The drawing under review shows one solid part. Ordinate dimensions are in mm from its lowest x, y, z. A direction names the side the tool comes from. Give positions to 0.01 mm unless a question says otherwise; leave off trailing zeros. Loops run counter-clockwise (first coordinate to the right, second up) from the corner with the lowest first, then second, coordinate; pieces in that order, holes last.
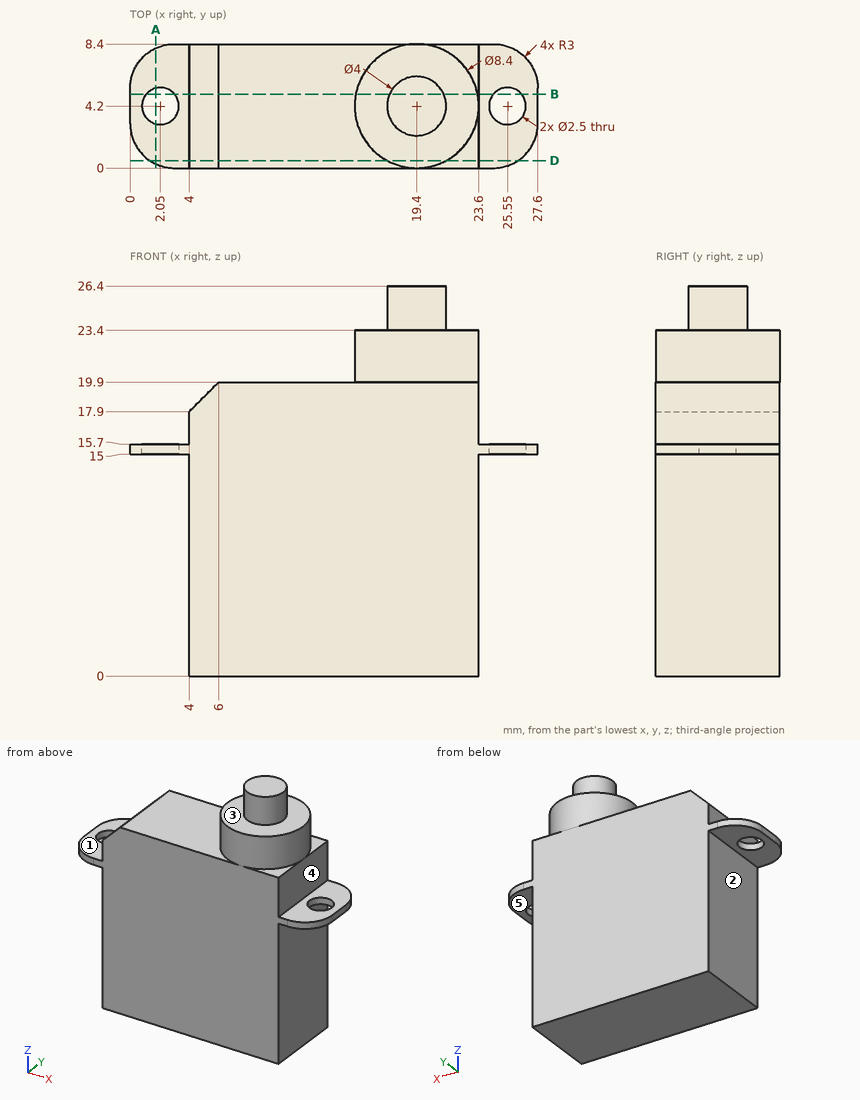
Item 1: Take a section at B-B on y = 5. State how many separate pieces and enclosed holes the cut face has, and give its area (3 significant figures).
Answer:
separate pieces: 3
enclosed holes: 0
area: 431 mm2
Item 2: For L1, parallel to Z at x = 23.5, y = 4.25; L2, parallel to Z at x = 11, y = 7.5; L3, parallel to Y at x = 2.05, z = 15.5, list the stretches that pass through material, from the lowest coordinate up.
Answer:
L1: z = 0 to 23.4
L2: z = 0 to 19.9
L3: y = 0.15 to 2.95, 5.45 to 8.25
Item 3: Tool access review of the marked faces 1, 2, 3, 4 and 5: name each direction out of +Z, -Z, +X, -X, +Y, -Y from which nothing blocks a thin tool from reaching the whole face with its end or side.
Answer:
face 1: +Z, -X, +Y, -Y
face 2: -Z, -X, +Y, -Y
face 3: +Z
face 4: +Z, +X, +Y, -Y
face 5: -Z, +X, +Y, -Y
Item 4: Take a section at A-A on x = 1.75. Give the boundary of the cut face in (y, z), and give its area (3 significant figures).
Answer:
outline: (0.27, 15) - (2.99, 15) - (2.99, 15.7) - (0.27, 15.7) - close; (5.41, 15) - (8.13, 15) - (8.13, 15.7) - (5.41, 15.7) - close
area: 3.80 mm2
Item 5: Clearance check with flat-ended pins moving along their axes: pin 1 Ø1.5 at (y, z) = (2, 22.5) entering from +X; pin 2 Ø3 at (x, y) = (1, 5) entering from -Z; pin 3 Ø1.2 at (x, y) = (25.5, 4.5) entering from -Z; pin 4 Ø2.5 at (y, z) = (4, 8.5) entering from -X. State where each tip first meets the part, or that it passes through.
Answer:
pin 1: stops at x = 23.34
pin 2: stops at z = 15
pin 3: passes through
pin 4: stops at x = 4
Item 6: Take a section at D-D on y = 0.5. Give the boundary of the cut face in (x, z), and give its area (3 significant figures).
Answer:
outline: (1.34, 15) - (4, 15) - (4, 0) - (23.6, 0) - (23.6, 15) - (26.26, 15) - (26.26, 15.7) - (23.6, 15.7) - (23.6, 19.9) - (21.39, 19.9) - (21.39, 23.4) - (17.41, 23.4) - (17.41, 19.9) - (6, 19.9) - (4, 17.9) - (4, 15.7) - (1.34, 15.7) - close
area: 406 mm2
